Here's how the part is built. I have some questions about the finished solid (model axes, mm). A direction names the side the tool comes from. Give positions to 0.01 mm unless a question says otherwise; leave off trailing zeros. Write each loop counter-clockwise with the first axis right and the second up, starting at its lowest first coordinate (ties: lowest second). Pieces come first, ordered by that corner, then holes. Notation, with made-up numbers: (42.25, 65.5) - (47.25, 65.5) arc R23 cw to (47.25, 93.5) - close; hole circle Ø10 at (47.25, 62.25). An arc over 180 degrees is marked (long way). One line per item, written item: value. Start each with the question number.
1) We'd pull the mould along X, two halves only. Please class faces 4 (the cylindrical face through (-87.07, -0.15, 3.23)), 5 (the flat face through (96, 1, 0)), 6 (the flat face through (-14, 11, 0)): +X half, -X half, draft (parallel to the pull), parting line (faces both ways), or undercut.
2) Imagine slicing it at C-C on x = 80.5. Write out the boundary of the cut face in (y, z), plus the area to 3 significant figures.
3) Please list where these lines run through material, in increasing order: L1, parallel to X at y = 0, z = -3.25; L2, parallel to X at y = 8.75, z = -12; L3, parallel to X at y = -4.75, z = 10. Write a range as [from, to].
4) I'm going to push a flat-ended pin straight in: P1, Ø5, axis at x = 36, y = 5, coming from the +Z side. Where does the tip first touch, or does it pass through?
5) On a 3-axis mill with a long thin cutter (end or side, diameter ignored), from which of +Z, -Z, +X, -X, +Y, -Y can I reach the whole of each face in a straight line? I mean faces 1 (the cylindrical face through (-43.65, 0.07, 8.11)), 2 (the flat face through (80, 7, 0)), 3 (the cylindrical face through (33, 5, 0)). Say none if no direction works.
6) Imagine slicing it at B-B on z = -14. Write out the boundary of the cut face in (x, y), plus the area to 3 significant figures.
7) Imagine slicing it at A-A on x = 36. Write out the boundary of the cut face in (y, z).
from build123d import *

# Parameters (mm, degrees)
SKETCH1_W                                        = 192
SKETCH1_H                                        = 22
BOSS_EXTRUDE1_DEPTH                              = 16
SKETCH3_W                                        = 25
SKETCH3_H                                        = 4
CUT_EXTRUDE4_DEPTH                               = 32
M12X1_5_TAPPED_HOLE5_D                           = 10.5
M12X1_5_TAPPED_HOLE5_DEPTH                       = 24
M12X1_5_TAPPED_HOLE5_CSINK_D                     = 12.05
M12X1_5_TAPPED_HOLE5_CSINK_ANGLE                 = 90
M12X1_5_TAPPED_HOLE5_TIP                         = 3.15451825
M4X0_7_TAPPED_HOLE1_D                            = 3.3
M4X0_7_TAPPED_HOLE1_DEPTH                        = 11.5
M4X0_7_TAPPED_HOLE1_CSINK_D                      = 4.05
M4X0_7_TAPPED_HOLE1_CSINK_ANGLE                  = 90
M4X0_7_TAPPED_HOLE1_TIP                          = 0.991420021
SKETCH18_R                                       = 3
CUT_EXTRUDE5_DEPTH                               = 102.788997441
CHAMFER1_SIZE                                    = 2
CSK_FOR_M10_FLAT_HEAD_MACHINE_SCREW2_D           = 6.5
CSK_FOR_M10_FLAT_HEAD_MACHINE_SCREW2_CSINK_D     = 13
CSK_FOR_M10_FLAT_HEAD_MACHINE_SCREW2_CSINK_ANGLE = 90
SKETCH24_R                                       = 3
CUT_EXTRUDE6_DEPTH                               = 100.779757466


# Read off the part's stored shape, not the designer's step: CSK for M4 Countersunk Flat Head Screw2, M4 Tapped Hole2
with BuildPart() as part:
    # Sketch1 → Boss-Extrude1 (new, symmetric)
    with BuildSketch(Plane.XY):
        Rectangle(SKETCH1_W, SKETCH1_H)
    extrude(amount=BOSS_EXTRUDE1_DEPTH, both=True)

    # Sketch3 → Cut-Extrude4 (cut)
    with BuildSketch(Plane.XY.offset(16)):
        with Locations((80.5, 9)):
            Rectangle(SKETCH3_W, SKETCH3_H)
    extrude(amount=-CUT_EXTRUDE4_DEPTH, mode=Mode.SUBTRACT)

    # M12x1.5 Tapped Hole5
    with Locations(Plane.XY.offset(16)):
        with Locations((12, 0), (-62, 0)):
            CounterSinkHole(M12X1_5_TAPPED_HOLE5_D / 2, M12X1_5_TAPPED_HOLE5_CSINK_D / 2, depth=M12X1_5_TAPPED_HOLE5_DEPTH, counter_sink_angle=M12X1_5_TAPPED_HOLE5_CSINK_ANGLE)
            with Locations((0, 0, -(M12X1_5_TAPPED_HOLE5_DEPTH + M12X1_5_TAPPED_HOLE5_TIP / 2))):  # 118° drill point
                Cone(0, M12X1_5_TAPPED_HOLE5_D / 2, M12X1_5_TAPPED_HOLE5_TIP, mode=Mode.SUBTRACT)

    # M4x0.7 Tapped Hole1
    with Locations(Plane.XZ.offset(11)):
        with Locations((-61.920151764, 4), (12.028225588, 4)):
            CounterSinkHole(M4X0_7_TAPPED_HOLE1_D / 2, M4X0_7_TAPPED_HOLE1_CSINK_D / 2, depth=M4X0_7_TAPPED_HOLE1_DEPTH, counter_sink_angle=M4X0_7_TAPPED_HOLE1_CSINK_ANGLE)
            with Locations((0, 0, -(M4X0_7_TAPPED_HOLE1_DEPTH + M4X0_7_TAPPED_HOLE1_TIP / 2))):  # 118° drill point
                Cone(0, M4X0_7_TAPPED_HOLE1_D / 2, M4X0_7_TAPPED_HOLE1_TIP, mode=Mode.SUBTRACT)

    # Sketch18 → Cut-Extrude5 (cut, through all)
    with BuildSketch(Plane.XY.offset(16)):
        with Locations((-38, 5)):
            Circle(SKETCH18_R)
        with Locations((36, 5)):
            Circle(SKETCH18_R)
    extrude(amount=-CUT_EXTRUDE5_DEPTH, mode=Mode.SUBTRACT)

    # Chamfer1
    chamfer1_edges = [part.edges().sort_by_distance(p)[0] for p in [
        (96, -11, 0),
        (-96, -11, 0),
        (-96, 11, 0),
    ]]
    chamfer(chamfer1_edges, length=CHAMFER1_SIZE)

    # CSK for M10 Flat Head Machine Screw2 (through all)
    with Locations(Plane.XZ.offset(11)):
        with Locations((80.5, 4)):
            CounterSinkHole(CSK_FOR_M10_FLAT_HEAD_MACHINE_SCREW2_D / 2, CSK_FOR_M10_FLAT_HEAD_MACHINE_SCREW2_CSINK_D / 2, counter_sink_angle=CSK_FOR_M10_FLAT_HEAD_MACHINE_SCREW2_CSINK_ANGLE)

    # Sketch24 → Cut-Extrude6 (cut, through all)
    with BuildSketch(Plane.XZ.offset(11)):
        with Locations(Location((-85.920151764, 6, 0), (0, 0, 270))):
            Circle(SKETCH24_R)
    extrude(amount=-CUT_EXTRUDE6_DEPTH, mode=Mode.SUBTRACT)

    # CSK for M4 Countersunk Flat Head Scr 2 → CSK for M4 Countersunk Flat Head Screw2 (revolve, cut)
    with BuildSketch(Plane(origin=(-86, 0, 0), x_dir=(1, 0, 0), z_dir=(0, -1, 0))):
        Polygon((0, 8.882881782), (0.75, 8.882881782), (0.75, 14.75), (2, 16), (0, 16), align=None)
        Polygon((0.75, -6), (0.75, 3.117108952), (0, 3.117108952), (0, -6.450645464), align=None)
    revolve(axis=Axis((-86, 0, 0), (0, 0, 1)), mode=Mode.SUBTRACT)

    # M4 Tapped Hole2 outline → M4 Tapped Hole2 (revolve, cut)
    with BuildSketch(Plane(origin=(-42, 0, 0), x_dir=(1, 0, 0), z_dir=(0, -1, 0))):
        Polygon((0, 16), (0, -0.991420021), (1.65, 0), (1.65, 16), align=None)
    revolve(axis=Axis((-42, 0, 0), (0, 0, 1)), mode=Mode.SUBTRACT)


solid = part.part
Numbers:
1. face 4: undercut
1. face 5: +X half
1. face 6: draft
2. outline: (-11, -16) - (7, -16) - (7, 0.75) - (-7.75, 0.75) - (-11, -2.5) - close; (-11, 10.5) - (-7.75, 7.25) - (7, 7.25) - (7, 16) - (-11, 16) - close
2. area: 448 mm^2
3. L1: [-96, -86.75], [-85.25, -67.25], [-56.75, 6.75], [17.25, 96]
3. L2: [-96, 68], [93, 96]
3. L3: [-96, -64.24], [-59.76, 9.76], [14.24, 96]
4. P1: through
5. face 1: +Z
5. face 2: +Z, -Z, +Y
5. face 3: +Z, -Z
6. outline: (-96, -9) - (-94, -11) - (94, -11) - (96, -9) - (96, 11) - (93, 11) - (93, 7) - (68, 7) - (68, 11) - (-94, 11) - (-96, 9) - close; hole circle Ø6 at (-38, 5); hole circle Ø6 at (36, 5)
6. area: 4,060 mm^2
7. outline: (-11, -16) - (2, -16) - (2, 16) - (-11, 16) - close; (8, -16) - (11, -16) - (11, 16) - (8, 16) - close
